Verification items for this drawing (mm, ordinates from the low corner). Round coordinates to 2 decimals unless told otherwise and drop trailing zeros. Order: outer loops, then holes, each group sorted by start corner. A loop starts at its lowest first (then second) coordinate and runs counter-clockwise, first axis right, second up.
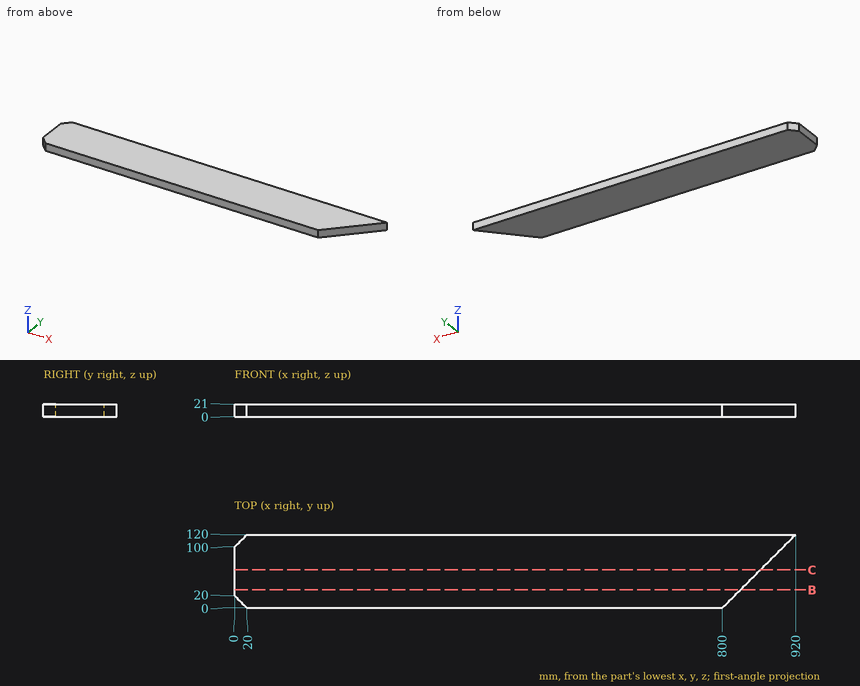
Item 1: Go/stop test with flat-tipped pins: P1, Ø3, axis at y = 38, z = 10.5, coming from the +X side; P2, Ø4, axis at y = 16, z = 6, coming from the +X side; P3, Ø5, axis at y = 92, z = 3.5, coming from the +X side. Record where each tip stops, or that it passes through.
Answer:
P1: stops at x = 839.5
P2: stops at x = 818
P3: stops at x = 894.5
Item 2: Sectioned sample at C-C (y = 62.5). Record the cut outline in (x, z).
Answer:
outline: (0, 0) - (862.5, 0) - (862.5, 21) - (0, 21) - close
Item 3: Scan lines: line 1 along X through (y, z) = (107, 8.25); line 2 along X through (y, z) = (71.5, 13.25); line 3 along Y through (x, z) = (853, 2.25). Record each from-to range of solid material in increasing order.
Answer:
line 1: x = 7 to 907
line 2: x = 0 to 871.5
line 3: y = 53 to 120
Item 4: Sectioned sample at B-B (y = 29.5). Record the cut outline in (x, z).
Answer:
outline: (0, 0) - (829.5, 0) - (829.5, 21) - (0, 21) - close
